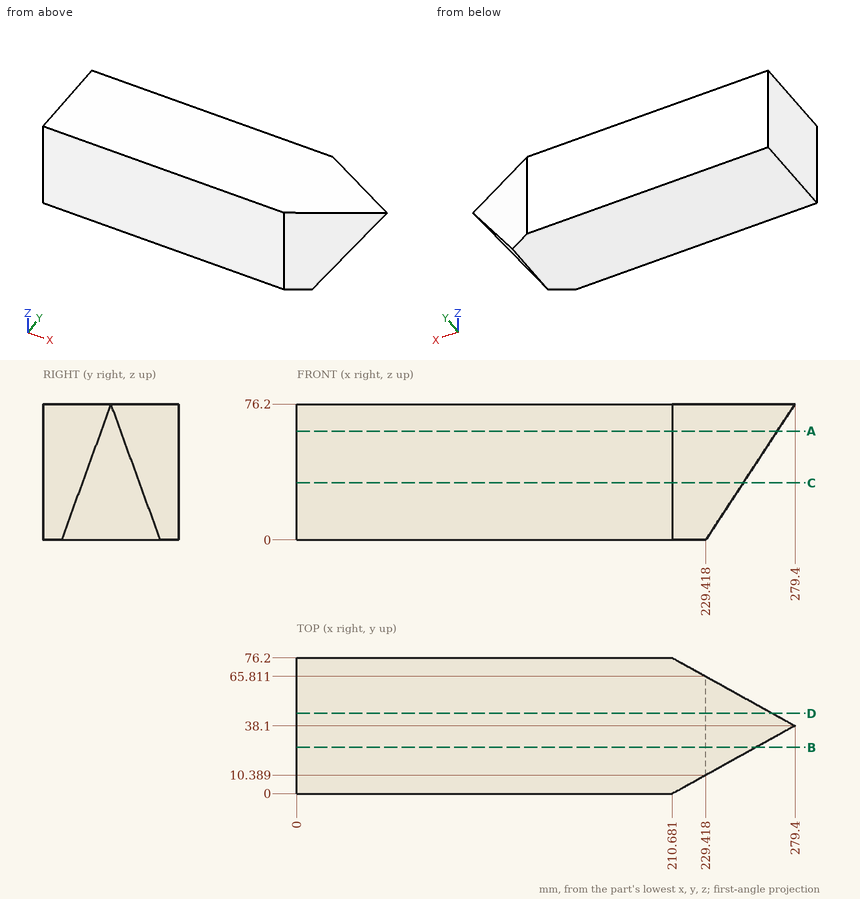
Verification items for this drawing (mm, ordinates from the low corner). Coordinates: 2 decimals unless noted, no trailing zeros. Order: outer loops, then holes, each group sorted by start corner. A loop starts at its lowest first (then second) coordinate and runs counter-clockwise, first axis right, second up. Notation, with made-up numbers: M 40,20 L 90,20 A6 ccw 90,26 Z; hole C 78.25,8.5 d2. An arc over 180 degrees is marked long. Write each question's results on one line, items separated by ' | '.
1) Section check C-C on z = 32. Record the cut outline in (x, y).
Solved:
outline: M 0,0 L 210.68,0 L 250.41,22.03 L 250.41,54.17 L 210.68,76.2 L 0,76.2 Z
2) Scan lines: line 1 along X through (y, z) = (27, 7); line 2 along X through (y, z) = (40, 43.5); line 3 along Z through (x, y) = (246, 30.5). Record each from-to range of solid material in increasing order. Write a range as [from, to].
Solved:
line 1: x = [0, 234.01] | line 2: x = [0, 257.95] | line 3: z = [25.28, 76.2]
3) Section check A-A on z = 61. Record the cut outline in (x, y).
Solved:
outline: M 0,0 L 210.68,0 L 269.43,32.57 L 269.43,43.63 L 210.68,76.2 L 0,76.2 Z
4) Section check D-D on y = 45. Record the cut outline in (x, z) (1 decimal).
Solved:
outline: M 0,0 L 229.4,0 L 267,57.2 L 267,76.2 L 0,76.2 Z
5) Gauge pin test, flat ends, axial feed: pin 1 Ø12 at (y, z) = (11.5, 53) entering from +X (1 decimal); pin 2 Ø1 at (y, z) = (14.5, 29.5) entering from +X (1 decimal); pin 3 Ø3 at (y, z) = (24.5, 8.5) entering from +X. Record the tip position at first contact, or that the pin passes through.
Solved:
pin 1: stops at x = 242.2 | pin 2: stops at x = 237.7 | pin 3: stops at x = 235.98
6) Section check B-B on y = 26. Record the cut outline in (x, z), plus the area to 3 significant figures.
Solved:
outline: M 0,0 L 229.42,0 L 257.58,42.93 L 257.58,76.2 L 0,76.2 Z | area: 19,000 mm²
